from build123d import *

# Parameters (mm, degrees)
ESTRUSIONE_ESTRUSIONE1_DEPTH = 30
SCHIZZO2_R                   = 1.5
ESTRUSIONE_ESTRUSIONE2_DEPTH = 7
FORO1_D                      = 2.459
FORO1_DEPTH                  = 7


with BuildPart() as part:
    # Schizzo1 → Estrusione-Estrusione1 (new body)
    with BuildSketch(Plane.XY):
        Polygon((1.25, -2.165063509), (2.5, 0), (1.25, 2.165063509), (-1.25, 2.165063509), (-2.5, 0), (-1.25, -2.165063509), align=None)
    extrude(amount=-ESTRUSIONE_ESTRUSIONE1_DEPTH)

    # Schizzo2 → Estrusione-Estrusione2 (add)
    with BuildSketch(Plane(origin=(0, 0, -30), x_dir=(-1, 0, 0), z_dir=(0, 0, -1))):
        Circle(SCHIZZO2_R)
    extrude(amount=ESTRUSIONE_ESTRUSIONE2_DEPTH)

    # Foro1
    with Locations(Plane.XY):
        with Locations((0, 0)):
            Hole(FORO1_D / 2, depth=FORO1_DEPTH)


solid = part.part
Could you check a few things on this model? Use its own coordinates, in mm. A direction names the side the tool comes from. Give positions to 0.01 mm unless a question says otherwise; leave off trailing zeros. Order: outer loops, then holes, each group sorted by start corner. A loop starts at its lowest first (then second) coordinate and runs counter-clockwise, first axis right, second up. Notation, with made-up numbers: (60, 36.5) - (86, 36.5) arc R8 cw to (86, 47.5) - close; hole circle Ø2 at (38.5, 39.5). An arc over 180 degrees is marked (long way). One line per item, written item: value. Start each with the question number.
1. Imagine slicing it at B-B on z = -22.5. List the corners of the cut face in (x, y) for me, plus the area to 3 significant figures.
2. Imagine slicing it at C-C on y = 0.35. List the corners of the cut face in (x, z) for me, plus the area to 3 significant figures.
3. For P1, Ø1.5, axis at x = 0, y = 0, coming from the +Z side, with a flat end and sliding along its axis, tell me the tip position at first contact or that it passes through.
4. Thinking about a two-plate mould opening in Y: for faces 4 (the face through (0, 0, -7)), 5 (the face through (0, -2.165, -15)), 6 (the face through (1.88, 1.07, -14.79)), which applies, +Y half, -Y half, draft (parallel to the pull), parting line (faces both ways), or undercut?
5. Imagine slicing it at D-D on x = -2. List the corners of the cut face in (y, z) for me.
6. Imagine slicing it at A-A on x = 0. List the corners of the cut face in (y, z) for me.
7. If I drill on probe 1 along Y at (x, z) = (0, -5); probe 2 along Z at (x, y) = (0.2, 1.9); probe 3 along Z at (x, y) = (1.1, -0.1), over which ranges is the centre line in solid material (lowest first)?
8. For faces 1 (the face through (1.866, -1.098, -14.79)), 2 (the face through (0.976, -0.748, -3.549)), 3 (the face through (1.5, 0.07, -33.45)), which set-ups out of +Z, -Z, +X, -X, +Y, -Y let a thin tool reach every point of the face, with its end or its side?
Values:
1. outline: (-2.5, 0) - (-1.25, -2.17) - (1.25, -2.17) - (2.5, 0) - (1.25, 2.17) - (-1.25, 2.17) - close
1. area: 16.2 mm²
2. outline: (-2.3, -30) - (-1.46, -30) - (-1.46, -37) - (1.46, -37) - (1.46, -30) - (2.3, -30) - (2.3, 0) - (1.18, 0) - (1.18, -7) - (-1.18, -7) - (-1.18, 0) - (-2.3, 0) - close
2. area: 142 mm²
3. P1: z = -7
4. face 4: undercut
4. face 5: -Y half
4. face 6: +Y half
5. outline: (-0.87, -30) - (0.87, -30) - (0.87, 0) - (-0.87, 0) - close
6. outline: (-2.17, -30) - (-1.5, -30) - (-1.5, -37) - (1.5, -37) - (1.5, -30) - (2.17, -30) - (2.17, 0) - (1.23, 0) - (1.23, -7) - (-1.23, -7) - (-1.23, 0) - (-2.17, 0) - close
7. probe 1: -2.17 to -1.23, 1.23 to 2.17
7. probe 2: -30 to 0
7. probe 3: -37 to -7
8. face 1: +Z, -Z, +X, -Y
8. face 2: +Z
8. face 3: -Z
